```python
from build123d import *

# Parameters (mm, degrees)
F0_R     = 3.306105
F1_DEPTH = 12.7
F2_R     = 2.534693
F3_DEPTH = 8.89


with BuildPart() as f1:
    # F0 (on Top) → F1 (new body)
    with BuildSketch(Plane.XY):
        with BuildLine():
            ThreePointArc((11.417595, -0.712938), (11.434271, -0.356642), (11.439832, 0))
            ThreePointArc((11.439832, 0), (11.432214, 0.417404), (11.409372, 0.834252))
            ThreePointArc((11.409372, 0.834252), (9.876647, 5.772486), (6.32622, 9.531458))
            ThreePointArc((6.32622, 9.531458), (5.667184, 9.937443), (4.982202, 10.297932))
            ThreePointArc((4.982202, 10.297932), (2.555693, 11.150703), (0, 11.439832))
            ThreePointArc((0, 11.439832), (-2.614917, 11.136963), (-5.091375, 10.244396))
            ThreePointArc((-5.091375, 10.244396), (-5.772486, 9.876647), (-6.42717, 9.46368))
            ThreePointArc((-6.42717, 9.46368), (-9.937443, 5.667184), (-11.417595, 0.712938))
            ThreePointArc((-11.417595, 0.712938), (-11.43967, -0.060796), (-11.409372, -0.834252))
            ThreePointArc((-11.409372, -0.834252), (-9.876647, -5.772486), (-6.32622, -9.531458))
            ThreePointArc((-6.32622, -9.531458), (-5.667184, -9.937443), (-4.982202, -10.297932))
            ThreePointArc((-4.982202, -10.297932), (0.060796, -11.43967), (5.091375, -10.244396))
            ThreePointArc((5.091375, -10.244396), (5.772486, -9.876647), (6.42717, -9.46368))
            ThreePointArc((6.42717, -9.46368), (9.937443, -5.667184), (11.417595, -0.712938))
        make_face()
        Circle(F0_R, mode=Mode.SUBTRACT)
        with BuildLine():
            ThreePointArc((6.32622, 9.531458), (9.876647, 5.772486), (11.409372, 0.834252))
            Line((11.409372, 0.834252), (16.56909, 9.566168))
            Line((16.56909, 9.566168), (6.32622, 9.531458))
        make_face()
        with BuildLine():
            Line((16.56909, -9.566168), (11.417595, -0.712938))
            ThreePointArc((11.417595, -0.712938), (9.937443, -5.667184), (6.42717, -9.46368))
            Line((6.42717, -9.46368), (16.56909, -9.566168))
        make_face()
        with BuildLine():
            ThreePointArc((0, 11.439832), (2.555693, 11.150703), (4.982202, 10.297932))
            Line((4.982202, 10.297932), (0, 19.132337))
            Line((0, 19.132337), (0, 11.439832))
        make_face()
        with BuildLine():
            Line((0, -19.132337), (5.091375, -10.244396))
            ThreePointArc((5.091375, -10.244396), (0.060796, -11.43967), (-4.982202, -10.297932))
            Line((-4.982202, -10.297932), (0, -19.132337))
        make_face()
        with BuildLine():
            ThreePointArc((-5.091375, 10.244396), (-2.614917, 11.136963), (0, 11.439832))
            Line((0, 11.439832), (0, 19.132337))
            Line((0, 19.132337), (-5.091375, 10.244396))
        make_face()
        with BuildLine():
            Line((-16.56909, -9.566168), (-6.32622, -9.531458))
            ThreePointArc((-6.32622, -9.531458), (-9.876647, -5.772486), (-11.409372, -0.834252))
            Line((-11.409372, -0.834252), (-16.56909, -9.566168))
        make_face()
        with BuildLine():
            ThreePointArc((-11.417595, 0.712938), (-9.937443, 5.667184), (-6.42717, 9.46368))
            Line((-6.42717, 9.46368), (-16.56909, 9.566168))
            Line((-16.56909, 9.566168), (-11.417595, 0.712938))
        make_face()
    extrude(amount=F1_DEPTH)

    # F2 (on face) → F3 (join)
    with BuildSketch(Plane.XY.offset(12.7)):
        with Locations((-5.170809, 5.042512)):
            Circle(F2_R)
    extrude(amount=F3_DEPTH)


solid = f1.part
```
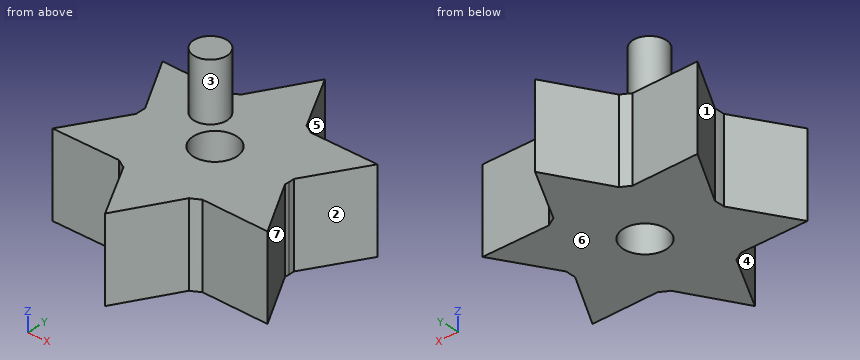
Geometry: final body of the model. Coordinates: model frame, mm. Face numbers are marked on the shaded views. A direction names the side the tool comes from. Round coordinates to 2 decimals unless told otherwise and drop trailing zeros. Write each loop counter-clockwise with the first axis right and the second up, starting at its lowest first coordinate (ties: lowest second). Pieces come first, ordered by that corner, then holes. Notation, with made-up numbers: (-28.75, 69.25) -> (-19.75, 69.25) arc R10 cw to (-19.75, 86.25) -> close; hole circle Ø2 at (84.5, -38). An arc over 180 degrees is marked (long way). Return JSON: item names as keys, results as strings.
Q1. Section D-D on y = -14. Return the cut outline in (x, z), and give its area (3 significant figures).
From the geometry:
{"outline": "(-2.89, 0) -> (2.94, 0) -> (2.94, 12.7) -> (-2.89, 12.7) -> close", "area": "74.1 mm2"}
Q2. Section A-A on x = 2. Return the cut outline in (y, z).
From the geometry:
{"outline": "(-15.64, 0) -> (-2.63, 0) -> (-2.63, 12.7) -> (-15.64, 12.7) -> close; (2.63, 0) -> (15.59, 0) -> (15.59, 12.7) -> (2.63, 12.7) -> close"}
Q3. Section B-B on y = 4.5. Return the cut outline in (x, z).
From the geometry:
{"outline": "(-13.62, 0) -> (13.58, 0) -> (13.58, 12.7) -> (-2.69, 12.7) -> (-2.69, 21.59) -> (-7.65, 21.59) -> (-7.65, 12.7) -> (-13.62, 12.7) -> close"}
Q4. Mould query, pull axis Y, two halves, no side actions, for the marked faces 4, 5, 6 and 7. Classes: +Y half, -Y half, draft (parallel to the pull), parting line (faces both ways), or undercut.
From the geometry:
{"face 4": "-Y half", "face 5": "+Y half", "face 6": "draft", "face 7": "undercut"}
Q5. Section C-C on z = 16.25. Return the cut outline in (x, y).
From the geometry:
{"outline": "circle Ø5.07 at (-5.17, 5.04)"}
Q6. Ray query, line 1 (X direction, y = 3, z = 11); line 2 (Y direction, x = -14.5, z = 1.75); line 3 (Z direction, x = 7.5, y = -9). Return the intervals inside material, ascending.
From the geometry:
{"line 1": "-12.75 to -1.39, 1.39 to 12.69", "line 2": "-9.56 to -6.06, 6.01 to 9.55", "line 3": "0 to 12.7"}
Q7. First-contact query: pin 1 Ø1.5 at (x, z) = (-12, 2.5) entering from +Y; pin 2 Ø7.5 at (x, y) = (0, 0) entering from +Z. Flat tips, straight axial feed; report the tip coordinate or a pass-through.
From the geometry:
{"pin 1": "y = 9.53", "pin 2": "z = 12.7"}
Q8. Set-up query: the marked faces 1, 2 and 3. Return all of +Z, -Z, +X, -X, +Y, -Y with unobstructed straight access to the full face (end or side cutting, diameter ignored); none if empty.
From the geometry:
{"face 1": "+Z, -Z, -X", "face 2": "+Z, -Z, +X", "face 3": "+Z"}
